```python
from build123d import *

# Parameters (mm, degrees)
SKETCH1_W           = 20
SKETCH1_H           = 19.85211399
BOSS_EXTRUDE1_DEPTH = 20
SKETCH2_R           = 7.5
CUT_EXTRUDE1_DEPTH  = 20
SKETCH3_R           = 7.5
BOSS_EXTRUDE2_DEPTH = 200


with BuildPart() as part:
    # Sketch1 → Boss-Extrude1 (new body)
    with BuildSketch(Plane(origin=(0, 0, 0), x_dir=(0, 0, -1), z_dir=(1, 0, 0))):
        with Locations((10, 9.926056995)):
            Rectangle(SKETCH1_W, SKETCH1_H)
    extrude(amount=BOSS_EXTRUDE1_DEPTH)

    # Sketch2 → Cut-Extrude1 (cut)
    with BuildSketch(Plane(origin=(0, 19.85211399, 0), x_dir=(1, 0, 0), z_dir=(0, 1, 0))):
        with Locations(Location((10, 10, 0), (0, 0, 270))):
            Circle(SKETCH2_R)
    extrude(amount=-CUT_EXTRUDE1_DEPTH, mode=Mode.SUBTRACT)

    # Sketch3 → Boss-Extrude2 (add)
    with BuildSketch(Plane(origin=(20, 0, 0), x_dir=(0, 0, -1), z_dir=(1, 0, 0))):
        with Locations((10, 9.926056995)):
            Circle(SKETCH3_R)
    extrude(amount=BOSS_EXTRUDE2_DEPTH)


solid = part.part
```
Can you work these out from the model? Positions are in its coordinate system, mm. Give positions to 0.01 mm unless a question says otherwise; leave off trailing zeros. Order: outer loops, then holes, each group sorted by start corner. A loop starts at its lowest first (then second) coordinate and runs counter-clockwise, first axis right, second up. Notation, with made-up numbers: (-33, 38.25) - (-12, 38.25) arc R23 ccw to (-12, 61.25) - close; hole circle Ø11 at (-15, 19). An arc over 180 degrees is marked (long way). Use a Markdown table: item, result. Add a question column.
Q1. If we section it at C-C on x = 125.5: Write out the boundary of the cut face in (y, z).
Q2. If we mould it in two halves opening along Z, with no side actions, what happens to faces 1 (the flat face through (10, 10, 0)), 2 (the cylindrical face through (2.68, 10.07, -11.63)), 3 (the cylindrical face through (118.6, 5.36, -4.05)), 4 (the flat face through (20, 17, -5))? For each: released by +Z, released by -Z, zero draft, split by the parting line, or undercut.
Q3. If we section it at A-A on x = 10: Write out the boundary of the cut face in (y, z), plus the area to 3 significant figures.
Q4. Please list where these lines run through material, in increasing order: line 1 along X through (y, z) = (12.5, -10); line 2 along Z through (x, y) = (9.5, 4); line 3 along Y through (x, z) = (203.5, -10.25).
Q5. I'm going to push flat-ended pins straight in: pin 1 (1 mm diameter, centred on x = 31.5, z = -10.5, fed in from +Y); pin 2 (12 mm diameter, centred on x = 130, z = -3, fed in from -Y); pin 3 (8 mm diameter, centred on x = 66.5, y = 13, fed in from -Z). Where does each tip first touch, or does it pass through?
Q6. If we section it at B-B on z = -10: Write out the boundary of the cut face in (x, y), plus the area to 3 significant figures.
Answers follow:
| question | item | result |
|---|---|---|
| 1 | outline | circle Ø15 at (9.93, -10) |
| 2 | face 1 | released by +Z |
| 2 | face 2 | undercut |
| 2 | face 3 | split by the parting line |
| 2 | face 4 | zero draft |
| 3 | outline | (0, -20) - (19.85, -20) - (19.85, -17.5) - (0, -17.5) - close; (0, -2.5) - (19.85, -2.5) - (19.85, 0) - (0, 0) - close |
| 3 | area | 99.3 mm^2 |
| 4 | line 1 | x = 0 to 2.5, 17.5 to 220 |
| 4 | line 2 | z = -20 to -17.48, -2.52 to 0 |
| 4 | line 3 | y = 2.43 to 17.42 |
| 5 | pin 1 | stops at y = 17.43 |
| 5 | pin 2 | stops at y = 2.49 |
| 5 | pin 3 | stops at z = -17.5 |
| 6 | outline | (0, 0) - (2.5, 0) - (2.5, 19.85) - (0, 19.85) - close; (17.5, 0) - (20, 0) - (20, 2.43) - (220, 2.43) - (220, 17.43) - (20, 17.43) - (20, 19.85) - (17.5, 19.85) - close |
| 6 | area | 3,100 mm^2 |
